The listing builds one solid part. Answer for the finished solid, in the listing's coordinates (mm). Face numbers are marked on the shaded views. A direction names the side the tool comes from. Round coordinates to 2 decimals unless told otherwise and drop trailing zeros. Loops run counter-clockwise (first coordinate to the right, second up) from the corner with the lowest first, then second, coordinate; pieces in that order, holes last. Notation, with made-up numbers: (52, -38.75) -> (71, -38.75) arc R14 ccw to (71, -26.75) -> close; hole circle Ø10 at (-14, 70.5). An arc over 180 degrees is marked (long way). Write each question's results on one line, items separated by ' | '. Start each with the question number.
Autodesk Inventor part; units mm, degrees
ref_plane "YZ Plane" through (0, 0, 0) normal (1, 0, 0) x (0, 1, 0)
ref_plane "XZ Plane" through (0, 0, 0) normal (0, 1, 0) x (-1, 0, 0)
ref_plane "XY Plane" through (0, 0, 0) normal (0, 0, 1) x (1, 0, 0)
sketch "Sketch1" plane through (0, 0, 0) normal (1, 0, 0) x (0, 1, 0)
  circle A0 centre (0, 0) radius 25
  line L0 (75, 75) -> (-75, 75)
  line L1 (-75, 75) -> (-75, -75)
  line L2 (-75, -75) -> (75, -75)
  line L3 (75, -75) -> (75, 75)
  dimension "d0" = 50
  dimension "d1" = 150
  dimension "d2" = 150
extrude "Extrusion1" add sketch "Sketch1" along normal blind 10 contours A0 | L3 L2 L1 L0
extrude "Extrusion2" add sketch "Sketch1" against normal blind 520 contours A0
fillet "Fillet1" radius 5 4 edges at (5, 75, -75) (5, 75, 75) (5, -75, -75) (5, -75, 75)
properties part number "Embolo"
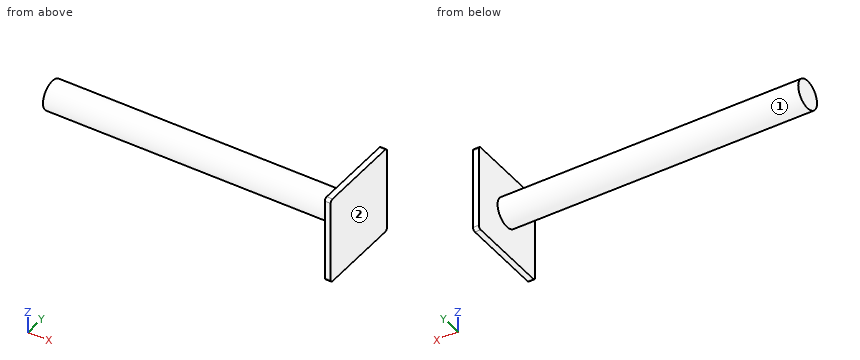
Item 1: The part is cut by section D-D, the plane z = -46. Give the vertices of the cut face in (x, y), plus the area to 3 significant figures.
Item 2: Straight lines are drawn through the part: L1, parallel to X at y = 14.5, z = -45.5; L2, parallel to Y at x = -444, z = -8.5; L3, parallel to Y at x = -121, z = -7. For each, find the intervals that lie inside material, in ascending order. Write a range as [from, to].
Item 3: Each of these flat-tipped pins is pushed along its axis until it touches: pin 1 Ø10 at (y, z) = (50.5, 54) entering from -X; pin 2 Ø1.5 at (x, y) = (-346, -2) entering from -Z; pin 3 Ø12 at (x, y) = (-254, 23) entering from +Z; pin 4 Ø4 at (x, y) = (-172.5, 28) entering from +Z. Where does it stop, or does it pass through?
Item 4: For the marked faces 1 and 2, determine the directions among +Z, -Z, +X, -X, +Y, -Y from which every point of the face is accessible in a straight line to the end or side of a thin tool.
Item 5: The part is cut by section C-C, the plane x = -364. Give the vertices of the cut face in (y, z), plus the area to 3 significant figures.
Item 6: The part is cut by section A-A, the plane y = 0. Give the vertices of the cut face in (x, z), plus the area to 3 significant figures.
Report:
1) outline: (0, -75) -> (10, -75) -> (10, 75) -> (0, 75) -> close | area: 1,500 mm2
2) L1: x = [0, 10] | L2: y = [-23.51, 23.51] | L3: y = [-24, 24]
3) pin 1: stops at x = 0 | pin 2: stops at z = -24.97 | pin 3: stops at z = 18.33 | pin 4: passes through
4) face 1: -X | face 2: +Z, -Z, +X, +Y, -Y
5) outline: circle Ø50 at (0, 0) | area: 1,960 mm2
6) outline: (-520, -25) -> (0, -25) -> (0, -75) -> (10, -75) -> (10, 75) -> (0, 75) -> (0, 25) -> (-520, 25) -> close | area: 27,500 mm2
